The model under review builds one solid part; all positions refer to its coordinate system, in mm. A direction names the side the tool comes from. Coordinates: 2 decimals unless noted, no trailing zeros. Loops run counter-clockwise (first coordinate to the right, second up) from the corner with the lowest first, then second, coordinate; pieces in that order, holes last. Notation, with made-up numbers: M 18,11.25 L 43,11.25 A22 cw 43,47.25 Z; hole C -15.75,61.25 d7. An arc over 180 degrees is marked long. One line per item, written item: value.
```python
from build123d import *

# Parameters (mm, degrees)
ESQUISSE1_W             = 52
ESQUISSE1_H             = 52
ESQUISSE1_W_2           = 42
ESQUISSE1_H_2           = 42
BOSS_EXTRU_1_DEPTH      = 11
ENL_V_START             = -53
ENL_V_MAT_EXTRU_1_DEPTH = 54
BOSS_EXTRU_2_DEPTH      = 2
BOSS_EXTRU_3_DEPTH      = 9
SYM_TRIE3_COPY_1_DEPTH  = 2
SYM_TRIE3_COPY_2_DEPTH  = 9
ENL_V_MAT_EXTRU_2_REACH = 54
ESQUISSE4_W             = 7
ESQUISSE4_H             = 8
ESQUISSE7_W             = 11
ESQUISSE7_H             = 6
BOSS_EXTRU_4_DEPTH      = 8
ENL_V_MAT_EXTRU_3_REACH = 62
ESQUISSE8_W             = 11
ESQUISSE8_H             = 1
ENL_V_MAT_EXTRU_4_DEPTH = 2.5
ESQUISSE10_R            = 2
ENL_V_MAT_EXTRU_5_DEPTH = 3.5


with BuildPart() as part:
    # Esquisse1 → Boss.-Extru.1 (new body)
    with BuildSketch(Plane.XY):
        Rectangle(ESQUISSE1_W, ESQUISSE1_H)
        Rectangle(ESQUISSE1_W_2, ESQUISSE1_H_2, mode=Mode.SUBTRACT)
    extrude(amount=BOSS_EXTRU_1_DEPTH)

    # Esquisse2 → Enlèv. mat.-Extru.1 (cut)
    with BuildSketch(Plane.ZY.offset(26).offset(ENL_V_START)):
        Polygon((88.428613369, 69.000029358), (11, 14.8), (9, 13.4), (9, 6.4), (11, 5), (88.428613369, -49.200029358), (277.455948436, -49.200029358), (277.455948436, 69.000029358), align=None)
    enl_v_mat_extru_1 = extrude(amount=ENL_V_MAT_EXTRU_1_DEPTH, mode=Mode.SUBTRACT)

    # Symétrie1: Enlèv. mat.-Extru.1 across plane
    add(enl_v_mat_extru_1.mirror(Plane.ZX), mode=Mode.SUBTRACT)

    # Esquisse3 → Boss.-Extru.2 (add)
    with BuildSketch(Plane.XY.offset(11)):
        Polygon((-21, 14.8), (-14.8, 21), (-21, 21), align=None)
    boss_extru_2 = extrude(amount=-BOSS_EXTRU_2_DEPTH)

    # Esquisse6 → Boss.-Extru.3 (add)
    with BuildSketch(Plane(origin=(0, 0, 9), x_dir=(-1, 0, 0), z_dir=(0, 0, -1))):
        Polygon((21, 21), (16.8, 21), (21, 16.8), align=None)
    boss_extru_3 = extrude(amount=BOSS_EXTRU_3_DEPTH)

    # Symétrie2: Boss.-Extru.2, Boss.-Extru.3 across plane
    add(boss_extru_2.mirror(Plane(origin=(0, 0, 0), x_dir=(0, 0, 1), z_dir=(1, 0, 0))))
    add(boss_extru_3.mirror(Plane(origin=(0, 0, 0), x_dir=(0, 0, 1), z_dir=(1, 0, 0))))

    # Symétrie3: Boss.-Extru.2, Boss.-Extru.3 across plane
    add(boss_extru_2.mirror(Plane.ZX))
    add(boss_extru_3.mirror(Plane.ZX))

    # Symétrie3 copy 1 sketch → Symétrie3 copy 1 (add)
    with BuildSketch(Plane(origin=(0, 0, 11), x_dir=(-1, 0, 0), z_dir=(0, 0, 1))):
        Polygon((-21, 14.8), (-14.8, 21), (-21, 21), align=None)
    extrude(amount=-SYM_TRIE3_COPY_1_DEPTH)

    # Symétrie3 copy 2 sketch → Symétrie3 copy 2 (add)
    with BuildSketch(Plane(origin=(0, 0, 9), x_dir=(1, 0, 0), z_dir=(0, 0, -1))):
        Polygon((21, 21), (16.8, 21), (21, 16.8), align=None)
    extrude(amount=SYM_TRIE3_COPY_2_DEPTH)

    # Esquisse4 → Enlèv. mat.-Extru.2 (cut, up to next)
    with BuildSketch(Plane.ZY.offset(26), mode=Mode.PRIVATE) as enl_v_mat_extru_2_sk1:
        with Locations((5.5, 0)):
            Rectangle(ESQUISSE4_W, ESQUISSE4_H)
    enl_v_mat_extru_2_tool1 = extrude(enl_v_mat_extru_2_sk1.sketch, amount=-ENL_V_MAT_EXTRU_2_REACH, mode=Mode.PRIVATE) & part.part
    add(enl_v_mat_extru_2_tool1.solids().sort_by_distance((-26, 0, 5.5))[0], mode=Mode.SUBTRACT)

    # Esquisse7 → Boss.-Extru.4 (add)
    with BuildSketch(Plane(origin=(26, 0, 0), x_dir=(0, 0, -1), z_dir=(1, 0, 0))):
        with Locations((-5.5, -1)):
            Rectangle(ESQUISSE7_W, ESQUISSE7_H)
    extrude(amount=BOSS_EXTRU_4_DEPTH)

    # Esquisse8 → Enlèv. mat.-Extru.3 (cut, up to next)
    with BuildSketch(Plane(origin=(34, 0, 0), x_dir=(0, 0, -1), z_dir=(1, 0, 0)), mode=Mode.PRIVATE) as enl_v_mat_extru_3_sk1:
        with Locations((-5.5, 0)):
            Rectangle(ESQUISSE8_W, ESQUISSE8_H)
    enl_v_mat_extru_3_tool1 = extrude(enl_v_mat_extru_3_sk1.sketch, amount=-ENL_V_MAT_EXTRU_3_REACH, mode=Mode.PRIVATE) & part.part
    add(enl_v_mat_extru_3_tool1.solids().sort_by_distance((34, 0, 5.5))[0], mode=Mode.SUBTRACT)

    # Esquisse9 → Enlèv. mat.-Extru.4 (cut)
    with BuildSketch(Plane.XZ.offset(4)):
        Polygon((33.464101615, 5.5), (31.732050808, 8.5), (28.267949192, 8.5), (26.535898385, 5.5), (28.267949192, 2.5), (31.732050808, 2.5), align=None)
    extrude(amount=-ENL_V_MAT_EXTRU_4_DEPTH, mode=Mode.SUBTRACT)

    # Esquisse10 → Enlèv. mat.-Extru.5 (cut)
    with BuildSketch(Plane.XZ.offset(1.5)):
        with Locations((30, 5.5)):
            Circle(ESQUISSE10_R)
    extrude(amount=-ENL_V_MAT_EXTRU_5_DEPTH, mode=Mode.SUBTRACT)


solid = part.part
```
(1) Add section B-B on y = -19. State the section outline as (x, z) points, then the cut area to 3 significant figures.
Checks:
outline: M -26,0 L -18.8,0 L -18.8,9 L -16.8,9 L -16.8,11 L -26,11 Z; M 16.8,9 L 18.8,9 L 18.8,0 L 26,0 L 26,11 L 16.8,11 Z
area: 166 mm^2
(2) Add section C-C on x = 30. State the section outline as (y, z) points, then the cut area to 3 significant figures.
Checks:
outline: M -4,0 L -0.5,0 L -0.5,3.5 L -1.5,3.5 L -1.5,2.5 L -4,2.5 Z; M -4,8.5 L -1.5,8.5 L -1.5,7.5 L -0.5,7.5 L -0.5,11 L -4,11 Z; M 0.5,0 L 2,0 L 2,3.5 L 0.5,3.5 Z; M 0.5,7.5 L 2,7.5 L 2,11 L 0.5,11 Z
area: 30.0 mm^2
(3) To check wall thickness, follow L1, parallel to Y at x = -10.5, z = 6; L2, parallel to Z at x = 30, y = -0.75. State the ranges of each line that lie inside material, in increasing order. Write a range as [from, to].
Checks:
L1: [-26, -21], [21, 26]
L2: [0, 3.5], [7.5, 11]
(4) Insertion check: pin 1 Ø1 at (y, z) = (7, 2) entering from +X; pin 2 Ø5.5 at (x, y) = (23.5, 9.5) entering from +Z; pin 3 Ø5.5 at (x, y) = (-24.5, -11) entering from +Z; pin 4 Ø3 at (x, z) = (30, 5.5) entering from +Y. Each pin has a flat end and moves straight along its axis. Give the tip position at first contact, or say it passes through.
Checks:
pin 1: x = 26
pin 2: z = 9
pin 3: z = 9.5
pin 4: through
(5) Add section D-D on x = 0.5. State the section outline as (y, z) points.
Checks:
outline: M -26,0 L -21,0 L -21,11 L -26,11 Z; M 21,0 L 26,0 L 26,11 L 21,11 Z
(6) Add section A-A on x = 20. State the section outline as (y, z) points, then the cut area to 3 significant figures.
Checks:
outline: M -26,0 L -17.8,0 L -17.8,9 L -15.8,9 L -15.8,11 L -26,11 Z; M 15.8,9 L 17.8,9 L 17.8,0 L 26,0 L 26,11 L 15.8,11 Z
area: 188 mm^2
(7) Tool access review of faces 1 (the face through (23.5, 14.1, 10)), 2 (the face through (32, 2, 4)), 3 (the face through (-24, 0, 2)), 4 (the face through (30, -3, 2.5)): name each direction out of +Z, -Z, +X, -X, +Y, -Y from which nothing blocks a thin tool from reaching the whole face with its end or side.
Checks:
face 1: +Z, +X, -X
face 2: +Z, -Z, +X, +Y
face 3: -X
face 4: -Y
(8) Draft analysis for pull direction Y (two halves, no side actions). For faces 5 (the face through (-24, -4, 5)), 6 (the face through (26, -15, 5)), 7 (the face through (30, -1.5, 8)), state which applies: pulls with the +Y half, pulls with the -Y half, needs draft (parallel to the pull), parting line crosses it, or undercut.
Checks:
face 5: undercut
face 6: needs draft
face 7: pulls with the -Y half
